from build123d import *

# Parameters (mm, degrees)
SKETCH1_W                                    = 40
SKETCH1_H                                    = 40
BOSS_EXTRUDE2_DEPTH                          = 2
SKETCH2_W                                    = 6
SKETCH2_H                                    = 4
BOSS_EXTRUDE5_DEPTH                          = 3
SKETCH4_R                                    = 3.5
SKETCH4_R_2                                  = 1.6
BOSS_EXTRUDE6_DEPTH                          = 4
MIRROR2_AT_THE_SECOND_PLANE_COPY_1_SKETC_W   = 6
MIRROR2_AT_THE_SECOND_PLANE_COPY_1_SKETC_H   = 4
MIRROR2_AT_THE_SECOND_PLANE_COPY_1_DEPTH     = 3
MIRROR2_AT_THE_SECOND_PLANE_COPY_2_SKETC_R   = 3.5
MIRROR2_AT_THE_SECOND_PLANE_COPY_2_SKETC_R_2 = 1.6
MIRROR2_AT_THE_SECOND_PLANE_COPY_2_DEPTH     = 4
CUT_EXTRUDE2_DEPTH                           = 2
SKETCH8_R                                    = 1.6
CUT_EXTRUDE3_DEPTH                           = 2
SKETCH18_W                                   = 6
SKETCH18_H                                   = 2
BOSS_EXTRUDE10_DEPTH                         = 32
SKETCH19_W                                   = 6
SKETCH19_H                                   = 2
BOSS_EXTRUDE11_DEPTH                         = 3
FILLET1_R                                    = 2


with BuildPart() as part:
    # Sketch1 → Boss-Extrude2 (new body)
    with BuildSketch(Plane.XY):
        Rectangle(SKETCH1_W, SKETCH1_H)
    extrude(amount=BOSS_EXTRUDE2_DEPTH)

    # Sketch2 → Boss-Extrude5 (add)
    with BuildSketch(Plane.XY.offset(2)):
        with Locations((-12, 10)):
            Rectangle(SKETCH2_W, SKETCH2_H)
    boss_extrude5 = extrude(amount=BOSS_EXTRUDE5_DEPTH)

    # Sketch4 → Boss-Extrude6 (add)
    with BuildSketch(Plane(origin=(0, 12, 0), x_dir=(1, 0, 0), z_dir=(0, 1, 0))):
        with Locations((-12, -6.6)):
            Circle(SKETCH4_R)
        with Locations(Location((-12, -6.6, 0), (0, 0, 270))):
            Circle(SKETCH4_R_2, mode=Mode.SUBTRACT)
    boss_extrude6 = extrude(amount=-BOSS_EXTRUDE6_DEPTH)

    # Mirror2: Boss-Extrude5, Boss-Extrude6 across plane
    add(boss_extrude5.mirror(Plane(origin=(0, 0, 0), x_dir=(0, 0, 1), z_dir=(1, 0, 0))))
    add(boss_extrude6.mirror(Plane(origin=(0, 0, 0), x_dir=(0, 0, 1), z_dir=(1, 0, 0))))

    # Mirror2 at the second plane: Boss-Extrude5, Boss-Extrude6 across plane
    add(boss_extrude5.mirror(Plane(origin=(0, 3, 0), x_dir=(0, 0, 1), z_dir=(0, -1, 0))))
    add(boss_extrude6.mirror(Plane(origin=(0, 3, 0), x_dir=(0, 0, 1), z_dir=(0, -1, 0))))

    # Mirror2 at the second plane copy 1 sketc → Mirror2 at the second plane copy 1 (add)
    with BuildSketch(Plane(origin=(0, 6, 2), x_dir=(-1, 0, 0), z_dir=(0, 0, 1))):
        with Locations((-12, 10)):
            Rectangle(MIRROR2_AT_THE_SECOND_PLANE_COPY_1_SKETC_W, MIRROR2_AT_THE_SECOND_PLANE_COPY_1_SKETC_H)
    extrude(amount=MIRROR2_AT_THE_SECOND_PLANE_COPY_1_DEPTH)

    # Mirror2 at the second plane copy 2 sketc → Mirror2 at the second plane copy 2 (add)
    with BuildSketch(Plane(origin=(0, -6, 0), x_dir=(-1, 0, 0), z_dir=(0, -1, 0))):
        with Locations((-12, -6.6)):
            Circle(MIRROR2_AT_THE_SECOND_PLANE_COPY_2_SKETC_R)
        with Locations(Location((-12, -6.6, 0), (0, 0, 270))):
            Circle(MIRROR2_AT_THE_SECOND_PLANE_COPY_2_SKETC_R_2, mode=Mode.SUBTRACT)
    extrude(amount=-MIRROR2_AT_THE_SECOND_PLANE_COPY_2_DEPTH)

    # Sketch7 → Cut-Extrude2 (cut)
    with BuildSketch(Plane.XY.offset(2)):
        with BuildLine():
            ThreePointArc((9.324585763, 1.324585763), (0, 3.8), (-9.324585763, 1.324585763))
            Line((-9.324585763, 1.324585763), (-11.657506391, 3.657506391))
            ThreePointArc((-11.657506391, 3.657506391), (0, 7), (11.657506391, 3.657506391))
            Line((11.657506391, 3.657506391), (9.324585763, 1.324585763))
        make_face()
    extrude(amount=-CUT_EXTRUDE2_DEPTH, mode=Mode.SUBTRACT)

    # Sketch8 → Cut-Extrude3 (cut)
    with BuildSketch(Plane(origin=(0, 0, 0), x_dir=(-1, 0, 0), z_dir=(0, 0, -1))):
        with Locations((0, -10)):
            Circle(SKETCH8_R)
    extrude(amount=-CUT_EXTRUDE3_DEPTH, mode=Mode.SUBTRACT)

    # Sketch18 → Boss-Extrude10 (add)
    with BuildSketch(Plane(origin=(0, 20, 0), x_dir=(1, 0, 0), z_dir=(0, 1, 0))):
        with Locations((17, -1)):
            Rectangle(SKETCH18_W, SKETCH18_H)
        with Locations((-17, -1)):
            Rectangle(SKETCH18_W, SKETCH18_H)
    extrude(amount=BOSS_EXTRUDE10_DEPTH)

    # Sketch19 → Boss-Extrude11 (add)
    with BuildSketch(Plane(origin=(0, 52, 0), x_dir=(1, 0, 0), z_dir=(0, 1, 0))):
        Polygon((20, 0), (-14, 0), (-14, -2), (-20, -2), (-20, -3.5), (20, -3.5), align=None)
        with Locations((-17, -1)):
            Rectangle(SKETCH19_W, SKETCH19_H)
    extrude(amount=-BOSS_EXTRUDE11_DEPTH)

    # Fillet1
    fillet1_edges = [part.edges().sort_by_distance(p)[0] for p in [
        (20, 52, 1.75),
        (14, 20, 1),
        (-20, 52, 1.75),
        (-14, 20, 1),
        (-14, 49, 1),
        (14, 49, 1),
        (20, -20, 1),
        (-20, -20, 1),
    ]]
    fillet(fillet1_edges, radius=FILLET1_R)


solid = part.part
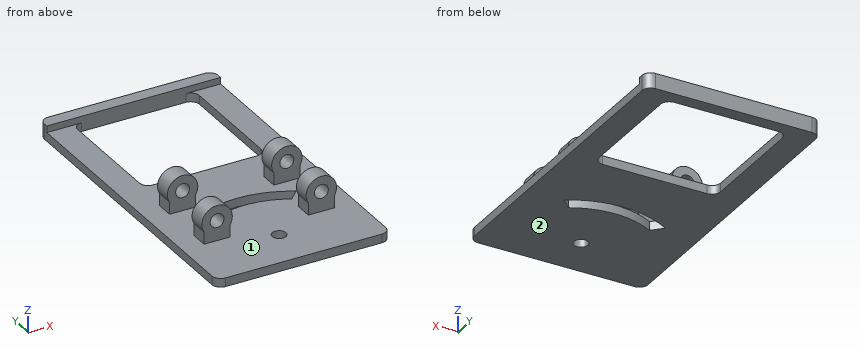
Can you work these out from the model? Positions are in its coordinate system, mm. Face numbers are marked on the shaded views. Round coordinates to 2 decimals unless told otherwise and drop trailing zeros. Loops run counter-clockwise (first coordinate to the right, second up) from the corner with the lowest first, then second, coordinate; pieces in that order, holes last. Notation, with made-up numbers: (56, 30.25) - (87, 30.25) arc R7 cw to (87, 40.25) - close; hole circle Ø10 at (34, -25.75). An arc over 180 degrees is marked (long way). Answer in a Markdown table with one row per item. Add a question column.
Q1. I want a section at A-A on y = -10. List the corners of the cut face in (x, z) for me, and give its area (3 significant figures).
Q2. I want a section at B-B on z = 6.6. Count the separate pieces of the cut face and the enclosed holes in it, and give its area (3 significant figures).
Q3. For pin 1 Ø3.5 at (x, z) = (-10.5, 7.5) entering from -Y; pin 2 Ø1.4 at (y, z) = (9, 3.5) entering from -X; pin 3 Ø3.5 at (x, y) = (8.5, 50) entering from +Z; pin 4 Ø3 at (x, z) = (12, 6.6) entering from -Y, each with a flat end and sliding along its axis, tell me the tip position at first contact or that it passes through.
Q4. I want a section at D-D on z = 1. List the corners of the cut face in (x, y) for me.
Q5. I need wall thicknesses on L1, parallel to X at y = -5, z = 6.6; L2, parallel to Y at x = 0, z = 1.5; L3, parallel to Y at x = -12.5, z = 9. Which ranges of each line are inside material? Lowest first, please.
Q6. I want a section at C-C on x = 0. List the corners of the cut face in (y, z) for me, and give its area (3 significant figures).
Q7. We'd pull the mould along Y, two halves only. Please class the marked faces 1 and 2: pulls with the +Y half, pulls with the -Y half, needs draft (parallel to the pull), parting line crosses it, or undercut.
A:
| question | item | result |
|---|---|---|
| 1 | outline | (-20, 0) - (-1.6, 0) - (-1.6, 2) - (-20, 2) - close; (1.6, 0) - (20, 0) - (20, 2) - (1.6, 2) - close |
| 1 | area | 73.6 mm^2 |
| 2 | separate pieces | 8 |
| 2 | enclosed holes | 0 |
| 2 | area | 60.8 mm^2 |
| 3 | pin 1 | y = -6 |
| 3 | pin 2 | x = -15 |
| 3 | pin 3 | z = 3.5 |
| 3 | pin 4 | through |
| 4 | outline | (-20, -18) arc R2 ccw to (-18, -20) - (18, -20) arc R2 ccw to (20, -18) - (20, 50) arc R2 ccw to (18, 52) - (-18, 52) arc R2 ccw to (-20, 50) - close; hole (-14, 22) arc R2 ccw to (-12, 20) - (12, 20) arc R2 ccw to (14, 22) - (14, 47) arc R2 ccw to (12, 49) - (-12, 49) arc R2 ccw to (-14, 47) - close; hole (-11.66, 3.66) - (-9.32, 1.32) arc R18.8 cw to (9.32, 1.32) - (11.66, 3.66) arc R22 ccw to start; hole circle Ø3.2 at (0, -10) |
| 5 | L1 | -15.5 to -13.6, -10.4 to -8.5, 8.5 to 10.4, 13.6 to 15.5 |
| 5 | L2 | -20 to -11.6, -8.4 to 3.8, 7 to 20, 49 to 52 |
| 5 | L3 | -6 to -2, 8 to 12 |
| 6 | outline | (-20, 0) - (-11.6, 0) - (-11.6, 2) - (-20, 2) - close; (-8.4, 0) - (3.8, 0) - (3.8, 2) - (-8.4, 2) - close; (7, 0) - (20, 0) - (20, 2) - (7, 2) - close; (49, 0) - (52, 0) - (52, 3.5) - (49, 3.5) - close |
| 6 | area | 77.7 mm^2 |
| 7 | face 1 | undercut |
| 7 | face 2 | needs draft |
